The figure shows three views and two pictorial views of one solid part (mm, origin at its lowest corner). Answer the questions. A direction names the side the tool comes from. Coordinates: 2 decimals unless noted, no trailing zeros. Write each loop counter-clockwise with the first axis right and the second up, starting at its lowest first coordinate (ties: lowest second). Pieces come first, ordered by that corner, then holes.
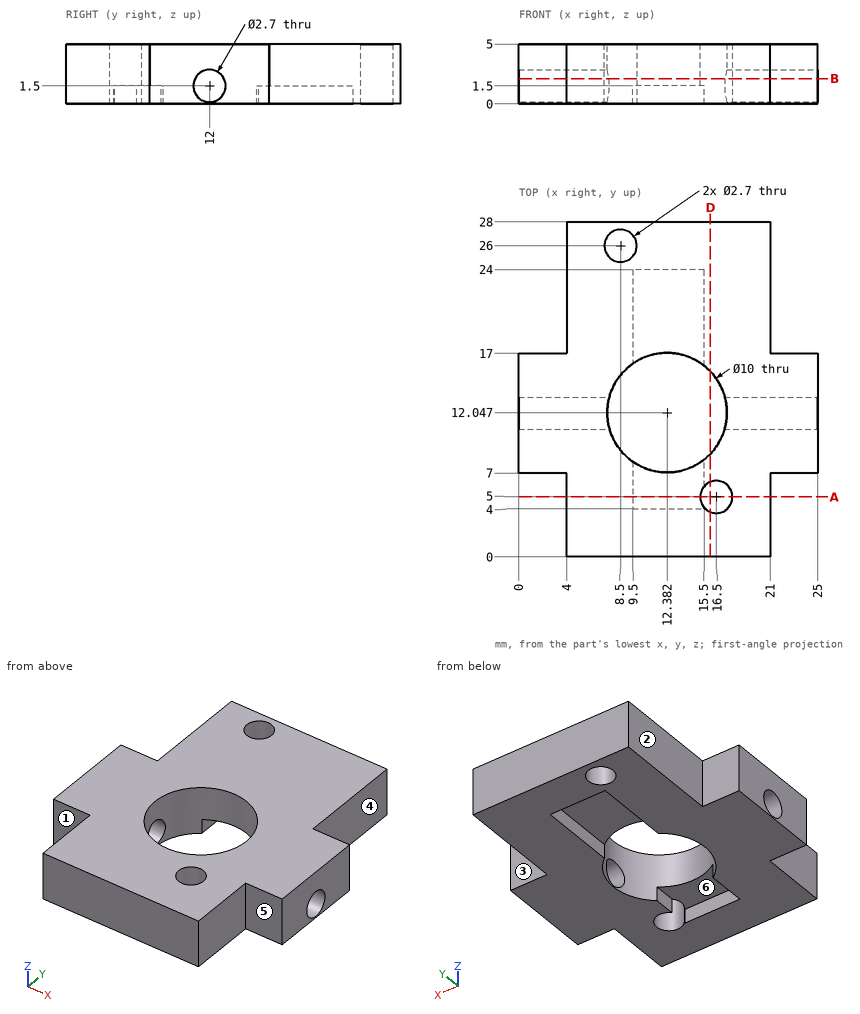
Q1. Find the intervals of material crossed by probe 1 along Y at (x, z) = (20.75, 1.5); probe 2 along Y at (x, z) = (13.25, 1.45); probe 3 along Z at (x, y) = (21.25, 12), in increasing order.
Answers below:
probe 1: y = 0 to 10.65, 13.35 to 28
probe 2: y = 0 to 4, 24 to 28
probe 3: z = 0 to 0.15, 2.85 to 5
Q2. The part is cut by section D-D, the plane x = 16. Write down the section's boundary in (y, z).
Answers below:
outline: (0, 0) - (3.75, 0) - (3.75, 5) - (0, 5) - close; (6.25, 0) - (8.6, 0) - (8.6, 5) - (6.25, 5) - close; (15.5, 0) - (28, 0) - (28, 5) - (15.5, 5) - close
Q3. Which of the six approach directions +Z, -Z, +X, -X, +Y, -Y give full straight-line access (tool end or side, diameter ignored) to the marked faces 1, 2 and 3?
Answers below:
face 1: +Z, -Z, -X, -Y
face 2: +Z, -Z, -X, +Y
face 3: +Z, -Z, +X, +Y
Q4. The part is cut by section B-B, the plane z = 2.1. State how many separate pieces and enclosed holes the cut face has.
Answers below:
separate pieces: 2
enclosed holes: 2
Q5. The part is cut by section A-A, the plane y = 5. Write down the section's boundary in (x, z).
Answers below:
outline: (4, 0) - (9.5, 0) - (9.5, 1.5) - (15.15, 1.5) - (15.15, 5) - (4, 5) - close; (17.85, 0) - (21, 0) - (21, 5) - (17.85, 5) - close
Q6. Determine the mould class of the marked faces 4, 5 and 6 for opening direction Y: released by +Y, released by -Y, zero draft, split by the parting line, or undercut.
Answers below:
face 4: zero draft
face 5: released by -Y
face 6: undercut
Q7. Given pin 1 (2.5 mm diameter, centred on y = 22, z = 2.5, fed in from +X); pin 2 (1.2 mm diameter, centred on y = 19, z = 0.5, fed in from -X); pin 3 (1.8 mm diameter, centred on x = 12.5, y = 19.5, fed in from -Z), each flat-ended and moving along its own axis, determine where each tip first touches the part or whether it passes through.
Answers below:
pin 1: stops at x = 21
pin 2: stops at x = 4
pin 3: stops at z = 1.5
